Geometry check sheet. Reference: the model listing, model coordinates, mm. A direction names the side the tool comes from. Coordinates: 2 decimals unless noted, no trailing zeros. Write each loop counter-clockwise with the first axis right and the second up, starting at its lowest first coordinate (ties: lowest second). Pieces come first, ordered by that corner, then holes. Notation, with made-up numbers: M 88.5,-34 L 133.5,-34 A13 cw 133.5,-25 Z; hole C -23,0.25 d11. An arc over 180 degrees is marked long. Put each result on its own line as item: value. Start each with the question number.
1) Scan lines: line 1 along X through (y, z) = (-6.7, 5); line 2 along X through (y, z) = (-9.6, 5); line 3 along Y through (x, z) = (10, -0.8). Record each from-to range of solid material in increasing order.
2) Gauge pin test, flat ends, axial feed: pin 1 (5 mm diameter, centred on x = -21.5, z = 4, fed in from -Y); pin 2 (10 mm diameter, centred on x = 12.5, y = -35.5, fed in from -Z); pin 3 (5 mm diameter, centred on x = -4.5, z = 6, fed in from -Y); pin 4 (1.9 mm diameter, centred on x = -22.5, z = 5, fed in from -Y). Record the tip position at first contact, or that the pin passes through.
3) Cross-section at D-D on x = -6. Record the cut outline in (y, z).
4) Mould release check, pull along X, two halves, no side actions. Record for faces 4 (the flat face through (25, -27, -1)), 5 (the flat face through (-12, -32, -2)), 6 (the flat face through (24, -32, -5)): released by +X, released by -X, zero draft, split by the parting line, or undercut.
5) Cross-section at B-B on z = 5. Record the cut outline in (x, y), plus the area to 3 significant figures.
6) Cross-section at A-A on x = 10. Record the cut outline in (y, z), plus the area to 3 significant figures.
7) Cross-section at C-C on y = -14. Record the cut outline in (x, z), plus the area to 3 significant figures.
8) Set-up check for faces 1 (the flat face through (-23, -7.951, 3)), 2 (the flat face through (0, -4.951, 4)), 3 (the flat face through (1.5, -32, -3)): record each of +Z, -Z, +X, -X, +Y, -Y from which the full face is reachable in a straight line by a thin tool's end or side.
from build123d import *

# Parameters (mm, degrees)
SKETCH_1_R          = 1.6
EXTRUDE_2_DEPTH     = 2
SKETCH_2_W          = 50
SKETCH_2_H          = 3
EXTRUDE_3_DEPTH     = 10
SKETCH_3_R          = 1.45
CUT_EXTRUDE_1_DEPTH = 3
EXTRUDE_4_DEPTH     = 50
SKETCH_8_R          = 1.6
CUT_EXTRUDE_4_DEPTH = 4
SKETCH_7_R          = 2.3
CUT_EXTRUDE_6_DEPTH = 20
SKETCH_10_W         = 3
SKETCH_10_H         = 55
EXTRUDE_5_DEPTH     = 3


with BuildPart() as part:
    # 草图1 → 凸台-拉伸2 (new body)
    with BuildSketch(Plane.XY):
        Polygon((25, -4.951489209), (25, -59.951489209), (-25, -59.951489209), (-25, -4.951489209), (0, -4.951489209), align=None)
        with Locations((10, -46.951489209)):
            Circle(SKETCH_1_R, mode=Mode.SUBTRACT)
        with Locations((-10, -46.951489209)):
            Circle(SKETCH_1_R, mode=Mode.SUBTRACT)
    extrude(amount=-EXTRUDE_2_DEPTH)

    # 草图2 → 凸台-拉伸3 (add)
    with BuildSketch(Plane.XY):
        with Locations((0, -6.451489209)):
            Rectangle(SKETCH_2_W, SKETCH_2_H)
    extrude(amount=EXTRUDE_3_DEPTH)

    # 草图3 → 切除-拉伸1 (cut)
    with BuildSketch(Plane(origin=(0, -7.951489209, 0), x_dir=(-1, 0, 0), z_dir=(0, -1, 0))):
        with Locations((22.5, -5)):
            Circle(SKETCH_3_R)
        with Locations((-22.5, -5)):
            Circle(SKETCH_3_R)
    extrude(amount=-CUT_EXTRUDE_1_DEPTH, mode=Mode.SUBTRACT)

    # 草图5 → 凸台-拉伸4 (add)
    with BuildSketch(Plane(origin=(25, -7.951489209, 0), x_dir=(0, 0, -1), z_dir=(1, 0, 0))):
        Polygon((-10, 0), (0, 0), (0, -5), align=None)
    extrude(amount=-EXTRUDE_4_DEPTH)

    # 草图8 → 切除-拉伸4 (cut, through all)
    with BuildSketch(Plane(origin=(0, -7.951489209, 0), x_dir=(-1, 0, 0), z_dir=(0, -1, 0))):
        with Locations((-22.5, -5)):
            Circle(SKETCH_8_R)
        with Locations((22.5, -5)):
            Circle(SKETCH_8_R)
    extrude(amount=-CUT_EXTRUDE_4_DEPTH, mode=Mode.SUBTRACT)

    # 草图7 → 切除-拉伸6 (cut)
    with BuildSketch(Plane(origin=(0, -7.951489209, 0), x_dir=(-1, 0, 0), z_dir=(0, -1, 0))):
        with Locations((-22.5, -5)):
            Circle(SKETCH_7_R)
        with Locations((22.5, -5)):
            Circle(SKETCH_7_R)
    extrude(amount=CUT_EXTRUDE_6_DEPTH, mode=Mode.SUBTRACT)

    # 草图10 → 凸台-拉伸5 (add)
    with BuildSketch(Plane(origin=(0, 0, -2), x_dir=(-1, 0, 0), z_dir=(0, 0, -1))):
        Polygon((-1.5, -59.951489209), (0, -59.951489209), (1.5, -59.951489209), (1.5, -4.951489209), (0, -4.951489209), (-1.5, -4.951489209), align=None)
        with Locations((23.5, -32.451489209)):
            Rectangle(SKETCH_10_W, SKETCH_10_H)
        with Locations((-23.5, -32.451489209)):
            Rectangle(SKETCH_10_W, SKETCH_10_H)
    extrude(amount=EXTRUDE_5_DEPTH)


solid = part.part
Answer key:
1. line 1: x = -25 to -24.1, -20.9 to 20.9, 24.1 to 25
1. line 2: x = -25 to -24.8, -20.2 to 20.2, 24.8 to 25
1. line 3: y = -59.95 to -48.55, -45.35 to -4.95
2. pin 1: stops at y = -12.2
2. pin 2: stops at z = -2
2. pin 3: stops at y = -11.2
2. pin 4: passes through
3. outline: M -59.95,-2 L -4.95,-2 L -4.95,10 L -7.95,10 L -12.95,0 L -59.95,0 Z
4. face 4: released by +X
4. face 5: undercut
4. face 6: zero draft
5. outline: M -25,-10.45 L -24.8,-10.45 L -24.8,-7.95 L -24.1,-7.95 L -24.1,-4.95 L -25,-4.95 Z; M -20.9,-7.95 L -20.2,-7.95 L -20.2,-10.45 L 20.2,-10.45 L 20.2,-7.95 L 20.9,-7.95 L 20.9,-4.95 L -20.9,-4.95 Z; M 24.1,-7.95 L 24.8,-7.95 L 24.8,-10.45 L 25,-10.45 L 25,-4.95 L 24.1,-4.95 Z
5. area: 233 mm²
6. outline: M -59.95,-2 L -48.55,-2 L -48.55,0 L -59.95,0 Z; M -45.35,-2 L -4.95,-2 L -4.95,10 L -7.95,10 L -12.95,0 L -45.35,0 Z
6. area: 159 mm²
7. outline: M -25,-5 L -22,-5 L -22,-2 L -1.5,-2 L -1.5,-5 L 1.5,-5 L 1.5,-2 L 22,-2 L 22,-5 L 25,-5 L 25,0 L -25,0 Z
7. area: 127 mm²
8. face 1: -Y
8. face 2: +Z, -Z, +X, -X, +Y
8. face 3: -Z, +Y, -Y
